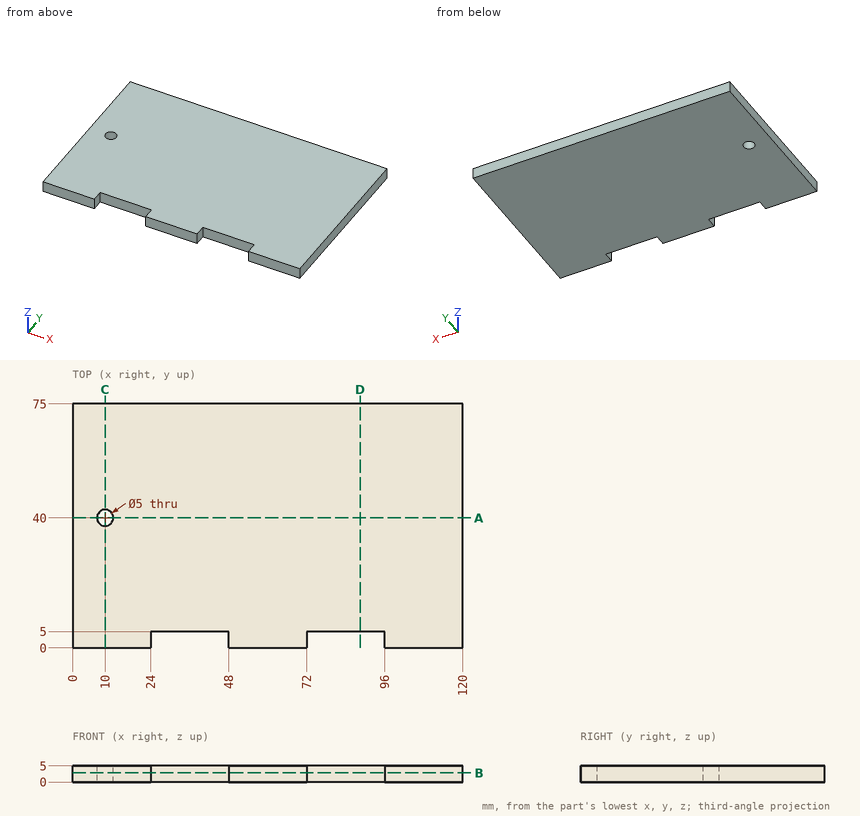
Source: three-view drawing plus pictorial views. Frame: mm from the lowest corner of the part. Give positions to 0.01 mm unless a question says otherwise; leave off trailing zeros. Order: outer loops, then holes, each group sorted by start corner. A loop starts at its lowest first (then second) coordinate and runs counter-clockwise, first axis right, second up. Notation, with made-up numbers: M 20,69 L 46,69 A16 ccw 46,87 Z; hole C 87,-12 d11. An arc over 180 degrees is marked long. One line per question, with ' | ' between items.
1) Section A-A on y = 40. Output: boundary loops of the cut face in (x, z), and give its area (3 significant figures).
Filled in:
outline: M 0,0 L 7.5,0 L 7.5,5 L 0,5 Z; M 12.5,0 L 120,0 L 120,5 L 12.5,5 Z | area: 575 mm2
2) Ray query, L1, parallel to Y at x = 10, z = 2.6; L2, parallel to Y at x = 43, z = 0.7. Return the intervals inside material, ascending.
Filled in:
L1: y = 0 to 37.5, 42.5 to 75 | L2: y = 5 to 75
3) Contact query for a flat-ended pin moving along its axis: P1, Ø2.5, axis at x = 38.5, z = 3, coming from the -Y side. Output: stop coordinate, or through.
Filled in:
P1: stops at y = 5
4) Section B-B on z = 2.8. Output: boundary loops of the cut face in (x, y), and give its area (3 significant figures).
Filled in:
outline: M 0,0 L 24,0 L 24,5 L 48,5 L 48,0 L 72,0 L 72,5 L 96,5 L 96,0 L 120,0 L 120,75 L 0,75 Z; hole C 10,40 d5 | area: 8,740 mm2
5) Section C-C on x = 10. Output: boundary loops of the cut face in (y, z), and give its area (3 significant figures).
Filled in:
outline: M 0,0 L 37.5,0 L 37.5,5 L 0,5 Z; M 42.5,0 L 75,0 L 75,5 L 42.5,5 Z | area: 350 mm2
6) Section D-D on x = 88.5. Output: boundary loops of the cut face in (y, z).
Filled in:
outline: M 5,0 L 75,0 L 75,5 L 5,5 Z
